from build123d import *

# Parameters (mm, degrees)
Y_KSEKLIK_EKSTR_ZYON1_DEPTH = 30
IZIM2_R                     = 7
IZIM2_R_2                   = 3.1
Y_KSEKLIK_EKSTR_ZYON2_DEPTH = 4
Y_KSEKLIK_EKSTR_ZYON3_START = 10
Y_KSEKLIK_EKSTR_ZYON3_DEPTH = 10
KES_EKSTR_ZYON2_START       = -10
KES_EKSTR_ZYON2_DEPTH       = 10
IZIM7_R                     = 1.75
KES_EKSTR_ZYON3_DEPTH       = 12


with BuildPart() as part:
    # Çizim1 → Yükseklik-Ekstrüzyon1 (new body)
    with BuildSketch(Plane(origin=(0, 0, 0), x_dir=(1, 0, 0), z_dir=(0, 1, 0))):
        with BuildLine():
            Line((-6.062177826, -3.5), (6.062177826, -3.5))
            ThreePointArc((6.062177826, -3.5), (0, 7), (-6.062177826, -3.5))
        make_face()
        with BuildLine():
            Line((-1.833030278, -2.5), (1.833030278, -2.5))
            ThreePointArc((1.833030278, -2.5), (0, 3.1), (-1.833030278, -2.5))
        make_face(mode=Mode.SUBTRACT)
    extrude(amount=Y_KSEKLIK_EKSTR_ZYON1_DEPTH)

    # Çizim2 → Yükseklik-Ekstrüzyon2 (add)
    with BuildSketch(Plane(origin=(0, 30, 0), x_dir=(1, 0, 0), z_dir=(0, 1, 0))):
        with Locations(Location((0, 0, 0), (0, 0, 210))):
            Circle(IZIM2_R)
        with Locations(Location((0, 0, 0), (0, 0, 233.750679117))):
            Circle(IZIM2_R_2, mode=Mode.SUBTRACT)
    extrude(amount=Y_KSEKLIK_EKSTR_ZYON2_DEPTH)

    # Çizim3 → Yükseklik-Ekstrüzyon3 (add)
    with BuildSketch(Plane.XZ.offset(Y_KSEKLIK_EKSTR_ZYON3_START)):
        with BuildLine():
            Line((-6.062177826, 3.5), (6.062177826, 3.5))
            ThreePointArc((6.062177826, 3.5), (0, -7), (-6.062177826, 3.5))
        make_face()
    extrude(amount=-Y_KSEKLIK_EKSTR_ZYON3_DEPTH)

    # Çizim5 → Kes-Ekstrüzyon2 (cut)
    with BuildSketch(Plane(origin=(0, 0, 0), x_dir=(1, 0, 0), z_dir=(0, 1, 0)).offset(KES_EKSTR_ZYON2_START)):
        with BuildLine():
            Line((-1.833030278, -2.5), (1.833030278, -2.5))
            ThreePointArc((1.833030278, -2.5), (0, 3.1), (-1.833030278, -2.5))
        make_face()
    extrude(amount=KES_EKSTR_ZYON2_DEPTH, mode=Mode.SUBTRACT)

    # Çizim7 → Kes-Ekstrüzyon3 (cut)
    with BuildSketch(Plane.XY.offset(3.5)):
        with Locations((0, -5)):
            Circle(IZIM7_R)
    extrude(amount=-KES_EKSTR_ZYON3_DEPTH, mode=Mode.SUBTRACT)


solid = part.part
Input: part model. Units: mm. Frame: model coordinates. A direction names the side the tool comes from. Coordinates: 2 decimals unless noted, no trailing zeros. Loops run counter-clockwise (first coordinate to the right, second up) from the corner with the lowest first, then second, coordinate; pieces in that order, holes last. Notation, with made-up numbers: (64, 37.25) -> (112, 37.25) arc R19 cw to (112, 69.25) -> close; hole circle Ø9 at (63.25, -30.5). An arc over 180 degrees is marked (long way). Write item = value, one per line. Start each with the question number.
Item 1: First-contact query: P1, Ø4, axis at y = -5.5, z = 3, coming from the -X side; P2, Ø1, axis at y = 25, z = -4.5, coming from the -X side; P3, Ø1.5, axis at y = 1.5, z = 3, coming from the +X side. Flat tips, straight axial feed; report the tip coordinate or a pass-through.
Item 2: Cut plane C-C, the plane y = -5. Return loops of the section in (x, z), plus the area to 3 significant figures.
Item 3: Material intervals for line 1 (Z direction, x = 0, y = 2); line 2 (X direction, y = 3.5, z = 0); line 3 (Y direction, x = 0, z = 3.05), sorted ascending.
Item 4: Mould query, pull axis Z, two halves, no side actions, for faces 1 (the face through (0, 10, 3.5)), 2 (the face through (-0.38, -6.71, 3.01)), 3 (the face through (-2.103, 11.692, -6.677)), 4 (the face through (0, 10, 2.5)). Classes: pulls with the +Z half, pulls with the -Z half, needs draft (parallel to the pull), parting line crosses it, or undercut.
Item 5: Reachability of faces 5 (the face through (0, 30, 5)), 6 (the face through (2, -10, -3)) from +Z, -Z, +X, -X, +Y, -Y: full face, straight path, thin tool, end or side. Return the list, or none.
Item 6: Cut plane D-D, the plane x = 3.5. Return loops of the section in (y, z).
Item 7: Cut plane B-B, the plane x = 0. Return loops of the section in (y, z), plus the area to 3 significant figures.
Item 8: Cut plane A-A, the plane z = 0. Return loops of the section in (x, y).
Ans:
q1.P1 = -6.93
q1.P2 = -5.74
q1.P3 = 6.63
q2.outline = (-6.06, 3.5) arc R7 ccw to (-1.75, -6.78) -> (-1.75, -2.56) arc R3.1 cw to (-1.83, 2.5) -> (-1.75, 2.5) -> (-1.75, 3.5) -> close; (1.75, -6.78) arc R7 ccw to (6.06, 3.5) -> (1.75, 3.5) -> (1.75, 2.5) -> (1.83, 2.5) arc R3.1 cw to (1.75, -2.56) -> close
q2.area = 77.6 mm²
q3.line_1 = -7 to -3.1, 2.5 to 3.5
q3.line_2 = -7 to -3.1, 3.1 to 7
q3.line_3 = -10 to -6.75, -3.25 to 30
q4.face_1 = pulls with the +Z half
q4.face_2 = needs draft
q4.face_3 = parting line crosses it
q4.face_4 = undercut
q5.face_5 = +Z, +X, -X, -Y
q5.face_6 = +Z, -Z, +X, -X, -Y
q6.outline = (-10, -6.06) -> (34, -6.06) -> (34, 6.06) -> (30, 6.06) -> (30, 3.5) -> (-10, 3.5) -> close
q7.outline = (-10, -7) -> (-6.75, -7) -> (-6.75, -3.1) -> (-10, -3.1) -> close; (-10, 2.5) -> (-6.75, 2.5) -> (-6.75, 3.5) -> (-10, 3.5) -> close; (-3.25, -7) -> (34, -7) -> (34, -3.1) -> (-3.25, -3.1) -> close; (-3.25, 2.5) -> (30, 2.5) -> (30, 3.1) -> (34, 3.1) -> (34, 7) -> (30, 7) -> (30, 3.5) -> (-3.25, 3.5) -> close
q7.area = 210 mm²
q8.outline = (-7, -10) -> (-3.1, -10) -> (-3.1, 34) -> (-7, 34) -> close; (3.1, -10) -> (7, -10) -> (7, 34) -> (3.1, 34) -> close
